from build123d import *

# Parameters (mm, degrees)
F0_R     = 12.5
F1_DEPTH = 32
F2_W     = 13
F2_H     = 31
F4_W     = 108.9288368821
F4_H     = 18.1096374691
F5_DEPTH = 65.001


with BuildPart() as f1:
    # F0 (on Top) → F1 (new body)
    with BuildSketch(Plane.XY):
        with BuildLine():
            ThreePointArc((0, 17.5), (5.1256313292, 5.1256313292), (17.5, 0))
            Line((17.5, 0), (102, 0))
            ThreePointArc((102, 0), (105.5355339059, 1.4644660941), (107, 5))
            Line((107, 5), (107, 60))
            ThreePointArc((107, 60), (105.5355339059, 63.5355339059), (102, 65))
            Line((102, 65), (5, 65))
            ThreePointArc((5, 65), (1.4644660941, 63.5355339059), (0, 60))
            Line((0, 60), (0, 17.5))
        make_face()
        with Locations((17.5, 17.5)):
            Circle(F0_R, mode=Mode.SUBTRACT)
    extrude(amount=F1_DEPTH)

    # F2 (on face) → F3 (revolve, cut)
    with BuildSketch(Plane.XY.offset(32)):
        with Locations((41.5, 17)):
            Rectangle(F2_W, F2_H)
        with Locations((59.5, 17)):
            Rectangle(F2_W, F2_H)
        with Locations((77.5, 17)):
            Rectangle(F2_W, F2_H)
        with Locations((95.5, 17)):
            Rectangle(F2_W, F2_H)
    revolve(axis=Axis((41.5, 32.5, 32), (1, 0, 0)), mode=Mode.SUBTRACT)

    # F4 (on face) → F5 (cut, through all)
    with BuildSketch(Plane.XZ):
        with Locations((54.4644184411, 27.0548187345)):
            Rectangle(F4_W, F4_H)
    extrude(amount=-F5_DEPTH, mode=Mode.SUBTRACT)


solid = f1.part
Geometry: final body of the model. Coordinates: model frame, mm. A direction names the side the tool comes from. Coordinates: 2 decimals unless noted, no trailing zeros. Loops run counter-clockwise (first coordinate to the right, second up) from the corner with the lowest first, then second, coordinate; pieces in that order, holes last. Notation, with made-up numbers: M 68,37.25 L 75,37.25 A19 ccw 75,69.25 Z; hole C 85.25,54 d2. An arc over 180 degrees is marked long. One line per item, written item: value. Start each with the question number.
1) Cut plane A-A (x = 20.5). Return loops of the section in (y, z).
2) Draft query along X for faces 1 (the flat face through (0, 39, 9)), 2 (the cylindrical face through (106, 63, 9)), 3 (the cylindrical face through (59.591, 32.022, 1.004)). Return one class per face: released by +X, released by -X, zero draft, split by the parting line, or undercut.
3) Cut plane B-B (z = 5). Return loops of the section in (x, y).
4) Cut plane D-D (y = 48). Return loops of the section in (x, z), then the cut area to 3 significant figures.
5) Reachability of faces 4 (the flat face through (107, 32, 9)), 5 (the flat face through (66, 33, 11)) from +Z, -Z, +X, -X, +Y, -Y: full face, straight path, thin tool, end or side. Return the list, or none.
6) Cut plane C-C (y = 12). Return loops of the section in (x, z).
7) Material intervals for L1, parallel to X at y = 42, z = 10; L2, parallel to Y at x = 17.5, z = 12.25; L3, parallel to X at y = 17.5, z = 5.75, sorted ascending. Write a range as from..to.
Evaluation:
1. outline: M 0,0 L 5.37,0 L 5.37,18 L 0,18 Z; M 29.63,0 L 65,0 L 65,18 L 29.63,18 Z
2. face 1: released by -X
2. face 2: released by +X
2. face 3: undercut
3. outline: M 0,17.5 A17.5 ccw 17.5,0 L 102,0 A5 ccw 107,5 L 107,60 A5 ccw 102,65 L 5,65 A5 ccw 0,60 Z; hole C 17.5,17.5 d25; hole M 35,17.27 L 48,17.27 L 48,47.73 L 35,47.73 Z; hole M 53,17.27 L 66,17.27 L 66,47.73 L 53,47.73 Z; hole M 71,17.27 L 84,17.27 L 84,47.73 L 71,47.73 Z; hole M 89,17.27 L 102,17.27 L 102,47.73 L 89,47.73 Z
4. outline: M 0,0 L 107,0 L 107,18 L 102,18 L 102,5.15 L 89,5.15 L 89,18 L 84,18 L 84,5.15 L 71,5.15 L 71,18 L 66,18 L 66,5.15 L 53,5.15 L 53,18 L 48,18 L 48,5.15 L 35,5.15 L 35,18 L 0,18 Z
4. area: 1,260 mm^2
5. face 4: +Z, -Z, +X, +Y, -Y
5. face 5: +Z
6. outline: M 0.89,0 L 6.28,0 L 6.28,18 L 0.89,18 Z; M 28.72,0 L 107,0 L 107,18 L 102,18 L 102,8.75 L 89,8.75 L 89,18 L 84,18 L 84,8.75 L 71,8.75 L 71,18 L 66,18 L 66,8.75 L 53,8.75 L 53,18 L 48,18 L 48,8.75 L 35,8.75 L 35,18 L 28.72,18 Z
7. L1: 0..35, 48..53, 66..71, 84..89, 102..107
7. L2: 0..5, 30..65
7. L3: 0..5, 30..35, 48..53, 66..71, 84..89, 102..107
